Design review of the part built by this model. Coordinates are the model's own, in mm. Face numbers are marked on the shaded views. Round coordinates to 2 decimals unless told otherwise and drop trailing zeros. Order: outer loops, then holes, each group sorted by start corner. A loop starts at its lowest first (then second) coordinate and runs counter-clockwise, first axis right, second up. Notation, with made-up numbers: (-11, -14.75) - (18, -14.75) arc R14 ccw to (18, -5.75) - close; hole circle Ø8 at (83, 8). An arc over 180 degrees is marked (long way). Use CSV: the item, a comma, the result in double quotes.
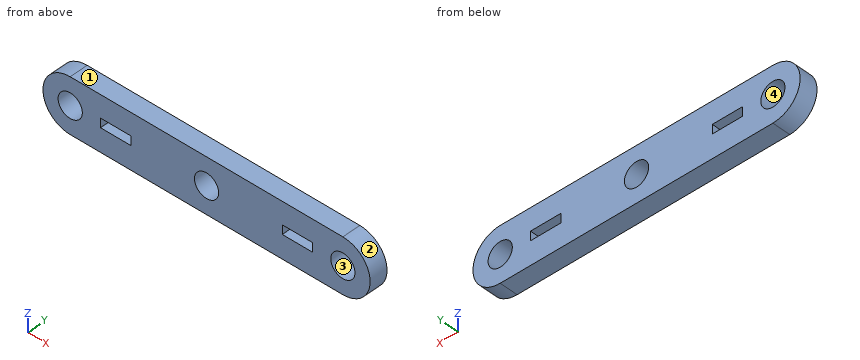
from build123d import *

# Parameters (mm, degrees)
BOSS_EXTRUDE1_DEPTH = 6
SKETCH3_R           = 4
CUT_EXTRUDE1_DEPTH  = 6
SKETCH4_W           = 10
SKETCH4_H           = 3
CUT_EXTRUDE2_DEPTH  = 6


with BuildPart() as part:
    # Sketch2 → Boss-Extrude1 (new body)
    with BuildSketch(Plane(origin=(0, 0, 0), x_dir=(1, 0, 0), z_dir=(0, 1, 0))):
        with BuildLine():
            Line((0, 0), (90, 0))
            ThreePointArc((90, 0), (99, 9), (90, 18))
            Line((90, 18), (0, 18))
            ThreePointArc((0, 18), (-9, 9), (0, 0))
        make_face()
    extrude(amount=BOSS_EXTRUDE1_DEPTH)

    # Sketch3 → Cut-Extrude1 (cut)
    with BuildSketch(Plane.XZ):
        with Locations(Location((0, -9, 0), (0, 0, 270))):
            Circle(SKETCH3_R)
        with Locations(Location((90, -9, 0), (0, 0, 90))):
            Circle(SKETCH3_R)
        with Locations(Location((45, -9, 0), (0, 0, 270))):
            Circle(SKETCH3_R)
    extrude(amount=-CUT_EXTRUDE1_DEPTH, mode=Mode.SUBTRACT)

    # Sketch4 → Cut-Extrude2 (cut)
    with BuildSketch(Plane(origin=(0, 6, 0), x_dir=(1, 0, 0), z_dir=(0, 1, 0))):
        with Locations((15, 8.821259453)):
            Rectangle(SKETCH4_W, SKETCH4_H)
        with Locations((75, 8.821259453)):
            Rectangle(SKETCH4_W, SKETCH4_H)
    extrude(amount=-CUT_EXTRUDE2_DEPTH, mode=Mode.SUBTRACT)


solid = part.part
1) We need section D-D (x = 45). Give the boundary of the cut face in (y, z), then the cut area to 3 significant figures.
Data:
outline,"(0, -18) - (6, -18) - (6, -13) - (0, -13) - close; (0, -5) - (6, -5) - (6, 0) - (0, 0) - close"
area,"60.0 mm2"
2) We need section C-C (y = 3.1). Give the boundary of the cut face in (x, z), then the cut area to 3 significant figures.
Data:
outline,"(0, -18) - (90, -18) arc R9 ccw to (90, 0) - (0, 0) arc R9 ccw to start; hole circle Ø8 at (0, -9); hole (10, -10.32) - (20, -10.32) - (20, -7.32) - (10, -7.32) - close; hole circle Ø8 at (45, -9); hole (70, -10.32) - (80, -10.32) - (80, -7.32) - (70, -7.32) - close; hole circle Ø8 at (90, -9)"
area,"1,660 mm2"
3) To check wall thickness, follow L1, parallel to X at y = 3.05, z = -9; L2, parallel to Z at x = 90, y = 3.2; L3, parallel to Z at x = 16, y = 1.9. State the ranges of each line that lie inside material, in increasing order. Write a range as from..to.
Data:
L1,"x = -9..-4, 4..10, 20..41, 49..70, 80..86, 94..99"
L2,"z = -18..-13, -5..0"
L3,"z = -18..-10.32, -7.32..0"
4) We need section A-A (x = 76). Give the boundary of the cut face in (y, z).
Data:
outline,"(0, -18) - (6, -18) - (6, -10.32) - (0, -10.32) - close; (0, -7.32) - (6, -7.32) - (6, 0) - (0, 0) - close"
5) Insertion check: pin 1 Ø3.5 at (y, z) = (2, -8.5) entering from +X. The pin has a flat end and moves straight along its axis. Give the tip position at first contact, or say it passes through.
Data:
pin 1,"stops at x = 99"
6) We need section B-B (z = -9). Give the boundary of the cut face in (x, y).
Data:
outline,"(-9, 0) - (-4, 0) - (-4, 6) - (-9, 6) - close; (4, 0) - (10, 0) - (10, 6) - (4, 6) - close; (20, 0) - (41, 0) - (41, 6) - (20, 6) - close; (49, 0) - (70, 0) - (70, 6) - (49, 6) - close; (80, 0) - (86, 0) - (86, 6) - (80, 6) - close; (94, 0) - (99, 0) - (99, 6) - (94, 6) - close"
7) The part is to be moulded in two halves that separate along Z. For the marked faces 1, 2, 3 and 4, say which applies: +Z half, -Z half, draft (parallel to the pull), parting line (faces both ways), or undercut.
Data:
face 1,"+Z half"
face 2,"parting line"
face 3,"undercut"
face 4,"undercut"
